For this review, take the finished solid that the model builds, in its own axes (mm). A direction names the side the tool comes from. Give positions to 0.01 mm unless a question says otherwise; leave off trailing zeros. Write each loop counter-clockwise with the first axis right and the second up, starting at its lowest first coordinate (ties: lowest second). Pieces come first, ordered by that corner, then holes.
Q1. Machinability: for faces 1 (the cylindrical face through (6.1, 1.5, -1.1)), 2 (the flat face through (2.55, 5, 0)), 3 (the flat face through (6, 19, 0)), 4 (the flat face through (6, 17, 2)), 5 (the flat face through (5.25, 1, 2)), which of the approach directions +Z, -Z, +X, -X, +Y, -Y give a long, thin tool a straight path to every point of the face, cutting with its end or side? Answer none if there is none.
Q2. We need section D-D (y = 15.64). Write out the cut boundary in (x, z), then the cut area to 3 significant figures.
Q3. We need section B-B (x = 4.75). Write out the cut boundary in (y, z).
Q4. Insertion check: P1, Ø0.8, axis at x = 8, z = 2.5, coming from the +Y side; P2, Ø1, axis at x = 8, y = 18, coming from the -Z side. Each pin has a flat end and moves straight along its axis. Give the tip position at first contact, or say it passes through.
Q5. For line 1 (Y direction, x = 3, z = 0.9); line 2 (Y direction, x = 8.8, z = 1.45); line 3 (X direction, y = 1.85, z = 0), list the stretches that pass through material, from the lowest coordinate up.
Q6. Mouldability with a two-part tool opening along Y and no side actions: class faces 6 (the cylindrical face through (9.349, 3.285, 0.033)), 7 (the flat face through (6, 17, -2)), 8 (the flat face through (6, 18, -1.75)) as released by +Y, released by -Y, zero draft, split by the parting line, or undercut.
Q7. We need section C-C (z = 0). Write out the cut boundary in (x, y), then the cut area to 3 significant figures.
Q8. We need section A-A (y = 5.25). Write out the cut boundary in (x, z).
```python
from build123d import *

# Parameters (mm, degrees)
F4_DEPTH  = 12.2
F6_W      = 8
F6_H      = 10
F7_DEPTH  = 5.5
F8_R      = 0.3
F9_DEPTH  = 5.501
F11_DEPTH = 3


with BuildPart() as f4:
    # F3 (on Right) → F4 (new body)
    with BuildSketch(Plane.YZ):
        Polygon((0, 2.35), (0, 0), (0, -2.35), (17, -2.35), (17, -1.75), (19, -1.75), (19, 0), (19, 1.75), (17, 1.75), (17, 2.35), align=None)
    extrude(amount=F4_DEPTH)

    # F6 (on offset) → F7 (join)
    with BuildSketch(Plane.XY.offset(2.75)):
        with Locations((6.1, 12)):
            Rectangle(F6_W, F6_H)
    extrude(amount=-F7_DEPTH)

    # F8 (on offset) → F9 (cut, through all)
    with BuildSketch(Plane.XY.offset(2.75)):
        with BuildLine():
            ThreePointArc((2.55, 4), (2.8428932188, 3.2928932188), (3.55, 3))
            Line((3.55, 3), (8.65, 3))
            ThreePointArc((8.65, 3), (9.3571067812, 3.2928932188), (9.65, 4))
            Line((9.65, 4), (9.65, 5.5))
            ThreePointArc((9.65, 5.5), (9.3571067812, 6.2071067812), (8.65, 6.5))
            Line((8.65, 6.5), (3.55, 6.5))
            ThreePointArc((3.55, 6.5), (2.8428932188, 6.2071067812), (2.55, 5.5))
            Line((2.55, 5.5), (2.55, 4))
        make_face()
        with Locations((2.8, 15.64)):
            Circle(F8_R)
        with Locations((8.8, 15.64)):
            Circle(F8_R)
    extrude(amount=-F9_DEPTH, mode=Mode.SUBTRACT)

    # F10 (on face) → F11 (cut, through all)
    with BuildSketch(Plane.XZ):
        with BuildLine():
            Line((6.95, 2.35), (5.25, 2.35))
            Line((5.25, 2.35), (5.25, 0.6982120022))
            ThreePointArc((5.25, 0.6982120022), (6.1, -1.1), (6.95, 0.6982120022))
            Line((6.95, 0.6982120022), (6.95, 2.35))
        make_face()
    extrude(amount=-F11_DEPTH, mode=Mode.SUBTRACT)


solid = f4.part
```
Computed:
1. face 1: -Y
1. face 2: +Z, -Z
1. face 3: +Z, -Z, +X, -X, +Y
1. face 4: +Z, +X, -X, +Y
1. face 5: +Z, -Y
2. outline: (0, -2.35) - (2.1, -2.35) - (2.1, -2.75) - (2.5, -2.75) - (2.5, 2.75) - (2.1, 2.75) - (2.1, 2.35) - (0, 2.35) - close; (3.1, -2.75) - (8.5, -2.75) - (8.5, 2.75) - (3.1, 2.75) - close; (9.1, -2.75) - (10.1, -2.75) - (10.1, -2.35) - (12.2, -2.35) - (12.2, 2.35) - (10.1, 2.35) - (10.1, 2.75) - (9.1, 2.75) - close
2. area: 57.1 mm2
3. outline: (0, -2.35) - (3, -2.35) - (3, 2.35) - (0, 2.35) - close; (6.5, -2.35) - (7, -2.35) - (7, -2.75) - (17, -2.75) - (17, -1.75) - (19, -1.75) - (19, 1.75) - (17, 1.75) - (17, 2.75) - (7, 2.75) - (7, 2.35) - (6.5, 2.35) - close
4. P1: stops at y = 17
4. P2: stops at z = -1.75
5. line 1: y = 0 to 3.16, 6.34 to 15.42, 15.86 to 19
5. line 2: y = 0 to 3.01, 6.49 to 15.34, 15.94 to 19
5. line 3: x = 0 to 5, 7.2 to 12.2
6. face 6: undercut
6. face 7: released by +Y
6. face 8: zero draft
7. outline: (0, 0) - (5, 0) - (5, 3) - (3.55, 3) arc R1 cw to (2.55, 4) - (2.55, 5.5) arc R1 cw to (3.55, 6.5) - (8.65, 6.5) arc R1 cw to (9.65, 5.5) - (9.65, 4) arc R1 cw to (8.65, 3) - (7.2, 3) - (7.2, 0) - (12.2, 0) - (12.2, 19) - (0, 19) - close; hole circle Ø0.6 at (2.8, 15.64); hole circle Ø0.6 at (8.8, 15.64)
7. area: 201 mm2
8. outline: (0, -2.35) - (2.55, -2.35) - (2.55, 2.35) - (0, 2.35) - close; (9.65, -2.35) - (12.2, -2.35) - (12.2, 2.35) - (9.65, 2.35) - close
